from build123d import *

# Parameters (mm, degrees)
PAD_DEPTH       = 150
SKETCH001_R     = 6
POCKET_DEPTH    = 18
SKETCH002_R     = 2
POCKET001_DEPTH = 2.001


with BuildPart() as part:
    # Sketch → Pad (new body)
    with BuildSketch(Plane.XY):
        with BuildLine():
            Line((0, 0), (-9.048751, 0))
            ThreePointArc((-9.048751, 0), (-9.737976, -0.275453), (-10.047503, -0.950062))
            Line((-10.047503, -0.950062), (-15, -100))
            Line((-15, -100), (-33, -100))
            Line((-33, -100), (-33, -97))
            ThreePointArc((-33, -97), (-34, -96), (-35, -97))
            Line((-35, -97), (-35, -101))
            ThreePointArc((-35, -101), (-34.707107, -101.707107), (-34, -102))
            Line((-34, -102), (0, -102))
            Line((0, -102), (0, 0))
        make_face()
    extrude(amount=PAD_DEPTH)

    # Sketch001 (on Face10 of Pad) → Pocket (cut)
    with BuildSketch(Plane(origin=(-20, 0, 0), x_dir=(0, -1, 0), z_dir=(-1, 0, 0))):
        with Locations((62, 30)):
            Circle(SKETCH001_R)
        with Locations((62, 120)):
            Circle(SKETCH001_R)
    extrude(amount=-POCKET_DEPTH, mode=Mode.SUBTRACT)

    # Sketch002 (on Face15 of Pocket) → Pocket001 (cut, through all)
    with BuildSketch(Plane(origin=(-2, 0, 0), x_dir=(0, -1, 0), z_dir=(-1, 0, 0))):
        with Locations((62, 120)):
            Circle(SKETCH002_R)
        with Locations((62, 30)):
            Circle(SKETCH002_R)
    extrude(amount=-POCKET001_DEPTH, mode=Mode.SUBTRACT)


solid = part.part
Check sheet for the modelled part. Datum: model origin and axes. Units: mm. A direction names the side the tool comes from. Round coordinates to 2 decimals unless told otherwise and drop trailing zeros. Loops run counter-clockwise (first coordinate to the right, second up) from the corner with the lowest first, then second, coordinate; pieces in that order, holes last. Notation, with made-up numbers: M -29,5.25 L -1,5.25 A21 ccw -1,14.25 Z; hole C 10,-2.5 d5. An arc over 180 degrees is marked long. One line per question, with ' | ' between items. Start each with the question number.
Item 1: Section check B-B (z = 120). Record the boundary of the cut face in (x, y), and give its area (3 significant figures).
Item 2: Section check C-C (x = -26). Record the boundary of the cut face in (y, z), and give its area (3 significant figures).
Item 3: Section check D-D (z = 51). Record the boundary of the cut face in (x, y), and give its area (3 significant figures).
Item 4: Scan lines: probe 1 along Z at (x, y) = (-9, -62); probe 2 along Z at (x, y) = (-0.4, -62); probe 3 along Y at (x, z) = (-6.75, 30). Record each from-to range of solid material in increasing order.
Item 5: Gauge pin test, flat ends, axial feed: pin 1 Ø9.5 at (y, z) = (-64.5, 31) entering from -X; pin 2 Ø13 at (y, z) = (-60.5, 119) entering from -X; pin 3 Ø5 at (y, z) = (-62, 120) entering from -X. Record the tip position at first contact, or that the pin passes through.
Item 6: Set-up check for faces 5 (the face through (-24, -100, 74)), 6 (the face through (-4, 0, 74)), 7 (the face through (-2, -62, 27)): record each of +Z, -Z, +X, -X, +Y, -Y from which the full face is reachable in a straight line by a thin tool's end or side.
Item 7: Release check for a two-part mould opening along Y. For faces 1 (the face through (-12.49, -49.78, 73.95)), 2 (the face through (-1, -62, 28)), 3 (the face through (-33, -99, 74)), 4 (the face through (-2, -65, 120)) record: released by +Y, released by -Y, zero draft, split by the parting line, or undercut.
Item 8: Section check A-A (y = -62). Record the boundary of the cut face in (x, z), and give its area (3 significant figures).
Worked out:
1) outline: M -35,-101 A1 ccw -34,-102 L 0,-102 L 0,-64 L -2,-64 L -2,-68 L -13.4,-68 L -15,-100 L -33,-100 L -33,-97 A1 ccw -35,-97 Z; M -12.8,-56 L -2,-56 L -2,-60 L 0,-60 L 0,0 L -9.05,0 A1 ccw -10.05,-0.95 Z | area: 1,190 mm^2
2) outline: M -102,0 L -100,0 L -100,150 L -102,150 Z | area: 300 mm^2
3) outline: M -35,-101 A1 ccw -34,-102 L 0,-102 L 0,0 L -9.05,0 A1 ccw -10.05,-0.95 L -15,-100 L -33,-100 L -33,-97 A1 ccw -35,-97 Z | area: 1,330 mm^2
4) probe 1: 0 to 24, 36 to 114, 126 to 150 | probe 2: 0 to 28, 32 to 118, 122 to 150 | probe 3: -102 to -68, -56 to 0
5) pin 1: x = -13.46 | pin 2: x = -13.3 | pin 3: x = -2
6) face 5: +Z, -Z, +Y | face 6: +Z, -Z, +X, -X, +Y | face 7: -X
7) face 1: released by +Y | face 2: undercut | face 3: zero draft | face 4: undercut
8) outline: M -13.1,0 L 0,0 L 0,28 L -2,28 L -2,24 L -13.1,24 Z; M -13.1,36 L -2,36 L -2,32 L 0,32 L 0,118 L -2,118 L -2,114 L -13.1,114 Z; M -13.1,126 L -2,126 L -2,122 L 0,122 L 0,150 L -13.1,150 Z | area: 1,680 mm^2
